```python
from build123d import *

# Parameters (mm, degrees)
F1_DEPTH  = 1870
F3_DEPTH  = 65.001
F5_DEPTH  = 125.001
F6_R      = 9
F7_DEPTH  = 7.5
F8_R      = 9
F9_DEPTH  = 7.5
F10_R     = 11
F11_DEPTH = 25


with BuildPart() as f1:
    # F0 (on Front) → F1 (new body)
    with BuildSketch(Plane.XZ):
        with BuildLine():
            Line((-25.16784, 62.5), (-25.16784, -62.5))
            Line((-25.16784, -62.5), (39.83216, -62.5))
            Line((39.83216, -62.5), (39.83216, -55))
            Line((39.83216, -55), (-12.46784, -55))
            ThreePointArc((-12.46784, -55), (-18.124695, -52.656854), (-20.46784, -47))
            Line((-20.46784, -47), (-20.46784, 47))
            ThreePointArc((-20.46784, 47), (-18.124695, 52.656854), (-12.46784, 55))
            Line((-12.46784, 55), (39.83216, 55))
            Line((39.83216, 55), (39.83216, 62.5))
            Line((39.83216, 62.5), (-25.16784, 62.5))
        make_face()
    extrude(amount=F1_DEPTH)

    # F2 (on face) → F3 (cut, through all)
    with BuildSketch(Plane(origin=(-25.16784, 0, 0), x_dir=(0, -1, 0), z_dir=(-1, 0, 0))):
        Polygon((125, 62.5), (0, 62.5), (0, -62.5), align=None)
    extrude(amount=-F3_DEPTH, mode=Mode.SUBTRACT)

    # F4 (on face) → F5 (cut, through all)
    with BuildSketch(Plane.XY.offset(62.5)):
        Polygon((-25.16784, -1870), (39.83216, -1870), (39.83216, -1805), align=None)
    extrude(amount=-F5_DEPTH, mode=Mode.SUBTRACT)

    # F6 (on face) → F7 (cut, through all)
    with BuildSketch(Plane.XY.offset(62.5)):
        with Locations((7.33216, -723)):
            Circle(F6_R)
        with Locations((7.33216, -825)):
            Circle(F6_R)
    extrude(amount=-F7_DEPTH, mode=Mode.SUBTRACT)

    # F8 (on face) → F9 (cut, through all)
    with BuildSketch(Plane.XY.offset(62.5)):
        with Locations((7.33216, -300)):
            Circle(F8_R)
        with Locations((7.33216, -402)):
            Circle(F8_R)
    extrude(amount=-F9_DEPTH, mode=Mode.SUBTRACT)

    # F10 (on face) → F11 (cut)
    with BuildSketch(Plane(origin=(-25.16784, 0, 0), x_dir=(0, -1, 0), z_dir=(-1, 0, 0))):
        with Locations((1832.5, 32.5)):
            Circle(F10_R)
        with Locations((1832.5, -32.5)):
            Circle(F10_R)
        with Locations((1171.5, 32.5)):
            Circle(F10_R)
        with Locations((1171.5, -32.5)):
            Circle(F10_R)
    extrude(amount=-F11_DEPTH, mode=Mode.SUBTRACT)


solid = f1.part
```
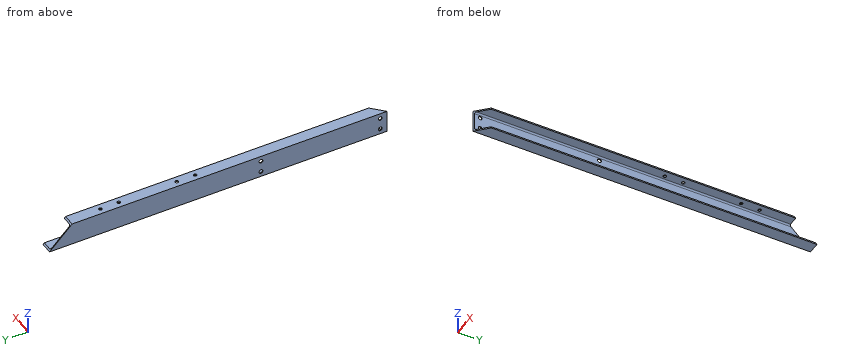
Geometry: final body of the model. Coordinates: model frame, mm. Coordinates: 2 decimals unless noted, no trailing zeros. Loops run counter-clockwise (first coordinate to the right, second up) from the corner with the lowest first, then second, coordinate; pieces in that order, holes last. Notation, with made-up numbers: M -20.5,-4 L 12.5,-4 A15 ccw 12.5,4 Z; hole C 8,-29.75 d5. An arc over 180 degrees is marked long. Put each result on its own line as item: value.
(1) Material intervals for probe 1 along Z at (x, y) = (-23, -1171); probe 2 along Z at (x, y) = (-7, -1678.5); probe 3 along X at (y, z) = (-723, 58.25), sorted ascending.
Answer sheet:
probe 1: z = -62.5 to -43.49, -21.51 to 21.51, 43.49 to 62.5
probe 2: z = -62.5 to -55, 55 to 62.5
probe 3: x = -25.17 to -1.67, 16.33 to 39.83
(2) First-contact query: pin 1 (16 mm diameter, centred on x = 7.33, y = -300, fed in from +Z). Flat tip, straight axial feed; report the tip coordinate or a pass-through.
Answer sheet:
pin 1: stops at z = -55
(3) Cut plane B-B on z = -4.5. Return the cut outline in (x, y).
Answer sheet:
outline: M -25.17,-1870 L -20.47,-1865.3 L -20.47,-58 L -25.17,-58 Z
(4) Cut plane A-A on y = -1510.5. Return the cut outline in (x, z), then the cut area to 3 significant figures.
Answer sheet:
outline: M -25.17,-62.5 L 39.83,-62.5 L 39.83,-55 L -12.47,-55 A8 cw -20.47,-47 L -20.47,47 A8 cw -12.47,55 L 39.83,55 L 39.83,62.5 L -25.17,62.5 Z
area: 1,520 mm^2
